Verification items for the finished model (mm, model axes). Face numbers are marked on the shaded views. A direction names the side the tool comes from. Round coordinates to 2 decimals unless told otherwise and drop trailing zeros. Write each loop counter-clockwise with the first axis right and the second up, starting at its lowest first coordinate (ties: lowest second). Pieces come first, ordered by that corner, then holes. Notation, with made-up numbers: (28.25, 36.5) -> (43.25, 36.5) arc R17 ccw to (43.25, 51.5) -> close; hole circle Ø2 at (69, -12.5). An arc over 180 degrees is marked (long way). Answer as a JSON object with one key per item and string values. Group by question number.
(1) Scan lines: L1, parallel to Z at x = 0, y = -2.5; L2, parallel to X at y = -5.75, z = 16; L3, parallel to Z at x = 27.5, y = -3.75. Record each from-to range of solid material in increasing order. Write a range as from..to.
(2) Set-up check for the marked faces 1, 2, 3 and 4: record each of +Z, -Z, +X, -X, +Y, -Y from which the full face is reachable in a straight line by a thin tool's end or side.
(3) Sectioned sample at A-A on z = 0. Record the cut outline in (x, y).
(4) Draft check along X on the marked faces 5, 6 and 7. Enter one of: released by +X, released by -X, zero draft, split by the parting line, or undercut.
(5) Sectioned sample at B-B on x = 0. Record the cut outline in (y, z).
(6) Gauge pin test, flat ends, axial feed: pin 1 Ø6 at (x, z) = (0, 0) entering from -Y; pin 2 Ø5 at (x, y) = (-4, -7) entering from +Z; pin 3 Ø8 at (x, z) = (12.5, -11) entering from +Y; pin 4 Ø5 at (y, z) = (-6, -3) entering from +X. Record the tip position at first contact, or that the pin passes through.
(7) Sectioned sample at D-D on z = -6. Record the cut outline in (x, y), and give its area (3 significant figures).
(8) Sectioned sample at C-C on y = -8.25. Record the cut outline in (x, z), and give its area (3 significant figures).
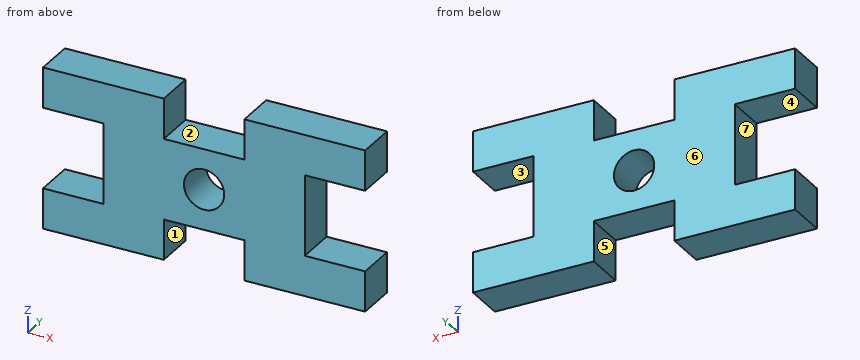
```python
from build123d import *

# Parameters (mm, degrees)
F0_R     = 5
F1_DEPTH = 10


with BuildPart() as f1:
    # F0 (on Front) → F1 (new body)
    with BuildSketch(Plane.XZ):
        Polygon((-10, -10), (0, -10), (10, -10), (10, -20), (40, -20), (40, -10), (25, -10), (25, 10), (40, 10), (40, 20), (10, 20), (10, 10), (0, 10), (-10, 10), (-10, 20), (-40, 20), (-40, 10), (-25, 10), (-25, -10), (-40, -10), (-40, -20), (-10, -20), align=None)
        Circle(F0_R, mode=Mode.SUBTRACT)
    extrude(amount=F1_DEPTH)


solid = f1.part
```
Computed values:
{
 "1": {"L1": "-10..-5, 5..10", "L2": "-40..-10, 10..40", "L3": "-20..-10, 10..20"},
 "2": {"face 1": "-Z, +Y, -Y", "face 2": "+Z, +Y, -Y", "face 3": "+X, +Y, -Y", "face 4": "-X, +Y, -Y"},
 "3": {"outline": "(-25, -10) -> (-5, -10) -> (-5, 0) -> (-25, 0) -> close; (5, -10) -> (25, -10) -> (25, 0) -> (5, 0) -> close"},
 "4": {"face 5": "undercut", "face 6": "zero draft", "face 7": "released by -X"},
 "5": {"outline": "(-10, -10) -> (0, -10) -> (0, -5) -> (-10, -5) -> close; (-10, 5) -> (0, 5) -> (0, 10) -> (-10, 10) -> close"},
 "6": {"pin 1": "through", "pin 2": "z = 10", "pin 3": "y = 0", "pin 4": "x = 25"},
 "7": {"outline": "(-25, -10) -> (25, -10) -> (25, 0) -> (-25, 0) -> close", "area": "500 mm2"},
 "8": {"outline": "(-40, -20) -> (-10, -20) -> (-10, -10) -> (10, -10) -> (10, -20) -> (40, -20) -> (40, -10) -> (25, -10) -> (25, 10) -> (40, 10) -> (40, 20) -> (10, 20) -> (10, 10) -> (-10, 10) -> (-10, 20) -> (-40, 20) -> (-40, 10) -> (-25, 10) -> (-25, -10) -> (-40, -10) -> close; hole circle Ø10 at (0, 0)", "area": "2,120 mm2"}
}
